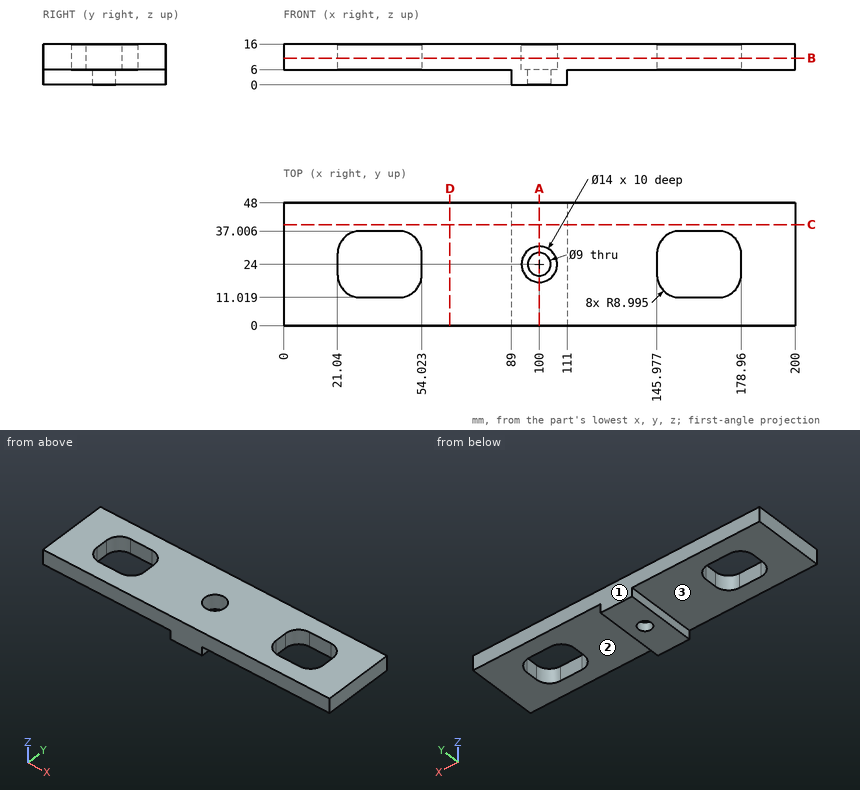
Verification items for this drawing (mm, ordinates from the low corner). A direction names the side the tool comes from. Coordinates: 2 decimals unless noted, no trailing zeros. Order: outer loops, then holes, each group sorted by start corner. A loop starts at its lowest first (then second) coordinate and runs counter-clockwise, first axis right, second up. Notation, with made-up numbers: (70.5, 20) -> (87.5, 20) arc R13 cw to (87.5, 25) -> close; hole circle Ø2 at (46, 88.25). An arc over 180 degrees is marked (long way). Put each result on its own line as item: value. Start each with the question number.
1. Cross-section at A-A, the plane x = 100. Record the boundary of the cut face in (y, z), then the cut area to 3 significant figures.
2. Cross-section at B-B, the plane z = 10.5. Record the boundary of the cut face in (x, y) (1 decimal), then the cut area to 3 significant figures.
3. Access from +Z, -Z, +X, -X, +Y, -Y to the whole of each face (thin tool, end or side, straight path). Record for the marked faces 1, 2 and 3.
4. Cross-section at D-D, the plane x = 65. Record the boundary of the cut face in (y, z).
5. Cross-section at C-C, the plane y = 39.5. Record the boundary of the cut face in (x, z), then the cut area to 3 significant figures.
6. Go/stop test with flat-tipped pins: pin 1 Ø6 at (x, z) = (125.5, 2) entering from +Y; pin 2 Ø12 at (x, y) = (106, 8.5) entering from -Z; pin 3 Ø7 at (x, y) = (103, 23.5) entering from +Z; pin 4 Ø3 at (y, z) = (15.5, 2.5) entering from +X. Record where each tip stops, or that it passes through.
7. Material ranges on L1, parallel to X at y = 24.5, z = 9; L2, parallel to Y at x = 100, z = 14; L3, parallel to Y at x = 100, z = 2.35, recorded low to high. Write a range as [from, to].
Computed:
1. outline: (0, 0) -> (19.5, 0) -> (19.5, 6) -> (17, 6) -> (17, 16) -> (0, 16) -> close; (28.5, 0) -> (48, 0) -> (48, 16) -> (31, 16) -> (31, 6) -> (28.5, 6) -> close
1. area: 574 mm2
2. outline: (0, 0) -> (200, 0) -> (200, 48) -> (0, 48) -> close; hole (21, 20) arc R9 ccw to (30, 11) -> (45, 11) arc R9 ccw to (54, 20) -> (54, 28) arc R9 ccw to (45, 37) -> (30, 37) arc R9 ccw to (21, 28) -> close; hole circle Ø14 at (100, 24); hole (146, 20) arc R9 ccw to (155, 11) -> (170, 11) arc R9 ccw to (179, 20) -> (179, 28) arc R9 ccw to (170, 37) -> (155, 37) arc R9 ccw to (146, 28) -> close
2. area: 7,870 mm2
3. face 1: +Z, -Z, +X, -X, +Y
3. face 2: -Z, +X, +Y, -Y
3. face 3: -Z, -X, +Y, -Y
4. outline: (0, 6) -> (48, 6) -> (48, 16) -> (0, 16) -> close
5. outline: (0, 6) -> (89, 6) -> (89, 0) -> (111, 0) -> (111, 6) -> (200, 6) -> (200, 16) -> (0, 16) -> close
5. area: 2,130 mm2
6. pin 1: through
6. pin 2: z = 0
6. pin 3: z = 6
6. pin 4: x = 111
7. L1: [0, 21.04], [54.02, 93.02], [106.98, 145.98], [178.96, 200]
7. L2: [0, 17], [31, 48]
7. L3: [0, 19.5], [28.5, 48]
